CAD build for the part. Positions are in the model's coordinates, mm. A direction names the side the tool comes from. Coordinates: 2 decimals unless noted, no trailing zeros. Write each loop counter-clockwise with the first axis right and the second up, starting at its lowest first coordinate (ties: lowest second). Pieces come first, ordered by that corner, then holes.
Autodesk Inventor part; units mm, degrees
ref_plane "YZ Plane" through (0, 0, 0) normal (1, 0, 0) x (0, 1, 0)
ref_plane "XZ Plane" through (0, 0, 0) normal (0, 1, 0) x (-1, 0, 0)
ref_plane "XY Plane" through (0, 0, 0) normal (0, 0, 1) x (1, 0, 0)
sketch "Sketch1" plane through (0, 0, 0) normal (0, 0, 1) x (1, 0, 0)
  point P0 (0, 0)
sketch "Sketch2" plane through (0, 0, 0) normal (1, 0, 0) x (0, 1, 0)
  line L0 (3.3322, 3.9709) -> (123.3322, 3.9709) construction
  line L1 (3.3322, 3.9709) -> (3.3322, -266.0291)
  line L2 (-116.6678, -266.0291) -> (3.3322, -266.0291)
  line L3 (3.3322, 3.9709) -> (-116.6678, -266.0291)
  point P0 (0, 0)
  dimension "d6" = 270
extrude "Extrusion1" add sketch "Sketch2" along normal blind 180
sketch "Sketch3" plane through (0, 3.3322, 3.9709) normal (0, 1, 0) x (1, 0, 0)
  line L0 (0, 0) -> (0, 270)
  line L1 (0, 270) -> (60, 270)
  line L2 (0, 270) -> (180, 270)
  line L3 (60, 270) -> (120, 270)
  line L4 (120, 270) -> (180, 270)
  line L5 (60, 270) -> (60, 195)
  line L6 (60, 195) -> (120, 195)
  line L7 (120, 195) -> (120, 270)
  point P0 (0, 3.9709)
  dimension "d7" = 60
  dimension "d8" = 60
  dimension "d9" = 75
extrude "Extrusion2" cut sketch "Sketch3" against normal blind 191.475
properties part number "Tapered"
Item 1: Saw through at A-A, the plane y = -91. Write the cut outline in (x, z).
Item 2: Two-plate mould, pull along X, no slides. Class faces 1 (the flat face through (88.74, -55.83, -129.14)), 2 (the flat face through (0, -31, -189)), 3 (the flat face through (90, -39, -191.029)): +X half, -X half, draft (parallel to the pull), parting line (faces both ways), or undercut.
Item 3: Saw through at D-D, the plane y = -69. Write the cut outline in (x, z), and give its area (3 significant figures).
Item 4: Wall check: line 1 along X through (y, z) = (-53.5, -245); line 2 along Z through (x, y) = (90, -11); line 3 along Z through (x, y) = (122, -72). Give the ranges that are in metal, low to high.
Item 5: Saw through at B-B, the plane z = -208.5. Write the cut outline in (x, y), and give its area (3 significant figures).
Item 6: Flat gauge pins, fed straight in: pin 1 Ø12 at (x, y) = (66.5, -37) entering from -Z; pin 2 Ø6 at (x, z) = (92, -74) entering from -Y. Where does each tip first touch, or does it go through?
Item 7: Saw through at C-C, the plane x = 44. Write the cut outline in (y, z).
Item 8: Which spindle directions (+Z, -Z, +X, -X, +Y, -Y) get a long thin tool onto all of the face, cutting with end or side? Do faces 4 (the flat face through (89, 3.332, -129)), 5 (the flat face through (120, -42, -228)). Say none if no direction does.
Working result:
1. outline: (0, -266.03) - (60, -266.03) - (60, -208.28) - (0, -208.28) - close; (120, -266.03) - (180, -266.03) - (180, -208.28) - (120, -208.28) - close
2. face 1: draft
2. face 2: -X half
2. face 3: undercut
3. outline: (0, -266.03) - (60, -266.03) - (60, -191.03) - (120, -191.03) - (120, -266.03) - (180, -266.03) - (180, -158.78) - (0, -158.78) - close
3. area: 14,800 mm2
4. line 1: x = 0 to 60, 120 to 180
4. line 2: z = -191.03 to -28.28
4. line 3: z = -266.03 to -165.53
5. outline: (0, -91.1) - (60, -91.1) - (60, 3.33) - (0, 3.33) - close; (120, -91.1) - (180, -91.1) - (180, 3.33) - (120, 3.33) - close
5. area: 11,300 mm2
6. pin 1: stops at z = -191.03
6. pin 2: stops at y = -32.65
7. outline: (-116.67, -266.03) - (3.33, -266.03) - (3.33, 3.97) - close
8. face 4: +Z, -Z, +X, -X, +Y
8. face 5: -Z, +Y, -Y
